Autodesk Inventor part; units mm, degrees
ref_plane "YZ Plane" through (0, 0, 0) normal (1, 0, 0) x (0, 1, 0)
ref_plane "XZ Plane" through (0, 0, 0) normal (0, 1, 0) x (-1, 0, 0)
ref_plane "XY Plane" through (0, 0, 0) normal (0, 0, 1) x (1, 0, 0)
sketch "Sketch1" plane through (0, 0, 0) normal (0, 1, 0) x (-1, 0, 0)
  circle A0 centre (0, 0) radius 20
  dimension "d0" = 40
extrude "Extrusion1" add sketch "Sketch1" along normal blind 152
fillet "Fillet1" radius 2 2 edges at (20, 152, 0) (20, 0, 0)
sketch "Sketch2" plane through (0, 0, 0) normal (0, -1, 0) x (1, 0, 0)
  circle A0 centre (0, 0) radius 7.5
  dimension "d4" = 15
extrude "Extrusion2" add sketch "Sketch2" along normal blind 30
properties part number "40152S" material "Lead"
Here's how the part is built. I have some questions about the finished solid (model axes, mm). A direction names the side the tool comes from. Coordinates: 2 decimals unless noted, no trailing zeros. Loops run counter-clockwise (first coordinate to the right, second up) from the corner with the lowest first, then second, coordinate; pieces in that order, holes last. Notation, with made-up numbers: (5, 81) -> (41, 81) arc R35 cw to (41, 117) -> close; hole circle Ø1 at (7.5, -25.5). An arc over 180 degrees is marked (long way). Use one line per item in the form item = value. Start each with the question number.
(1) If we section it at B-B (x = 0): Please give me the cut outline in (y, z).
(2) Will these pins go through, and if not, where does the flat tip stop? pin 1 (5 mm diameter, centred on y = 123.5, z = 15.5, fed in from -X); pin 2 (1.5 mm diameter, centred on x = 9, z = -15.5, fed in from -Y); pin 3 (10 mm diameter, centred on y = 87, z = 6.5, fed in from +X).
(3) On a 3-axis mill with a long thin cutter (end or side, diameter ignored), from which of +Z, -Z, +X, -X, +Y, -Y can I reach the whole of each face in a straight line? I mean faces 1 (the face through (0, 0, -8)), 2 (the face through (4.336, 74.964, 19.524)). Say none if no direction works.
(4) If we section it at A-A (z = 0): Please give me the cut outline in (x, y), then the cut area to 3 significant figures.
(5) If we section it at C-C (y = 87.5): Please give me the cut outline in (x, z).
(6) Please list where these lines run through material, in increasing order: line 1 along Y through (x, z) = (-11, -13); line 2 along Z through (x, y) = (1, 10); line 3 along X through (y, z) = (28.5, 9.5).
Verdict:
q1.outline = (-30, -7.5) -> (0, -7.5) -> (0, -18) arc R2 ccw to (2, -20) -> (150, -20) arc R2 ccw to (152, -18) -> (152, 18) arc R2 ccw to (150, 20) -> (2, 20) arc R2 ccw to (0, 18) -> (0, 7.5) -> (-30, 7.5) -> close
q2.pin_1 = -15.2
q2.pin_2 = 0
q2.pin_3 = 19.94
q3.face_1 = -Y
q3.face_2 = +Y, -Y
q4.outline = (-20, 2) arc R2 ccw to (-18, 0) -> (-7.5, 0) -> (-7.5, -30) -> (7.5, -30) -> (7.5, 0) -> (18, 0) arc R2 ccw to (20, 2) -> (20, 150) arc R2 ccw to (18, 152) -> (-18, 152) arc R2 ccw to (-20, 150) -> close
q4.area = 6,530 mm²
q5.outline = circle Ø40 at (0, 0)
q6.line_1 = 0 to 152
q6.line_2 = -19.97 to 19.97
q6.line_3 = -17.6 to 17.6
